from build123d import *

# Parameters (mm, degrees)
F1_DEPTH = 10
F2_R     = 1
F3_DEPTH = 6.2


# Not quite as in the source:
# - ends of sketch curves that miss each other by under 0.0002 mm in the source are joined


with BuildPart() as f1:
    # F0 (on Top) → F1 (new body)
    with BuildSketch(Plane.XY):
        with BuildLine():
            Line((-0.3999973293, 5), (-6.2999973293, 5))
            Line((-6.2999973293, 5), (-6.2999973293, -5))
            Line((-6.2999973293, -5), (6.3, -5))
            Line((6.3, -5), (6.3, 5))
            Line((6.3, 5), (0.4, 5))
            ThreePointArc((0.4, 5), (0.2585786438, 4.9414213562), (0.2, 4.8))
            Line((0.2, 4.8), (0.2, 0))
            ThreePointArc((0.2, 0), (0.1414213562, -0.1414213562), (0, -0.2))
            ThreePointArc((0, -0.2), (-0.1414186856, -0.1414213562), (-0.1999973293, 0))
            Line((-0.1999973293, 0), (-0.1999973293, 4.8))
            ThreePointArc((-0.1999973293, 4.8), (-0.2585759731, 4.9414213562), (-0.3999973293, 5))
        make_face()
    extrude(amount=F1_DEPTH)

    # F2 (on face) → F3 (cut)
    with BuildSketch(Plane(origin=(-6.2999973293, 0, 0), x_dir=(0, -1, 0), z_dir=(-1, 0, 0))):
        with Locations((-3, 5)):
            Circle(F2_R)
    extrude(amount=-F3_DEPTH, mode=Mode.SUBTRACT)


solid = f1.part
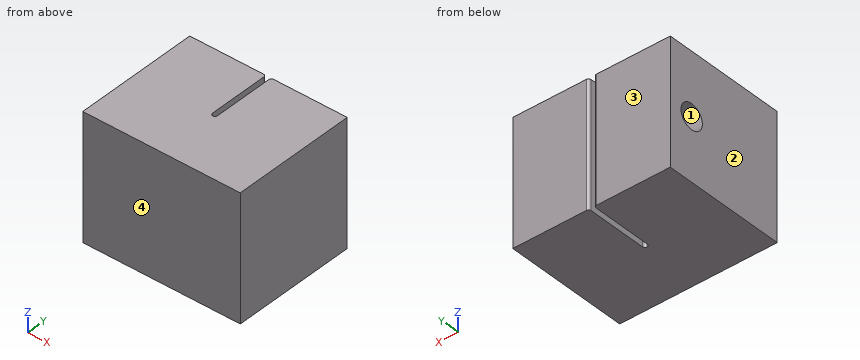
Could you check a few things on this model? Use its own coordinates, in mm. Face numbers are marked on the shaded views. Give positions to 0.01 mm unless a question says otherwise; leave off trailing zeros. Order: outer loops, then holes, each group sorted by start corner. A loop starts at its lowest first (then second) coordinate and runs counter-clockwise, first axis right, second up.
1. We'd pull the mould along Y, two halves only. Please class the marked faces 1, 2, 3 and 4: pulls with the +Y half, pulls with the -Y half, needs draft (parallel to the pull), parting line crosses it, or undercut.
2. I need wall thicknesses on L1, parallel to Z at x = -1.75, y = 3; L2, parallel to X at y = 2, z = 6; L3, parallel to X at y = 3.75, z = 4.75. Which ranges of each line are inside material? Lowest first, please.
3. Suppose I cut it at C-C (x = -1). List the corners of the cut face in (y, z) for me, plus the area to 3 significant figures.
4. Suppose I cut it at A-A (z = 5). List the corners of the cut face in (x, y) for me, plus the area to 3 significant figures.
5. Will these pins go through, and if not, where does the flat tip stop? P1, Ø1.6, axis at y = 3, z = 5, coming from the -X side; P2, Ø5, axis at y = 3, z = 5.5, coming from the -X side.
6. Suppose I cut it at B-B (y = 3). List the corners of the cut face in (x, z) for me, plus the area to 3 significant figures.
7. Suppose I cut it at D-D (z = 9). List the corners of the cut face in (x, y) for me.
Solved:
1. face 1: undercut
1. face 2: needs draft
1. face 3: pulls with the +Y half
1. face 4: pulls with the -Y half
2. L1: z = 0 to 4, 6 to 10
2. L2: x = -6.3 to -0.2, 0.2 to 6.3
2. L3: x = 0.2 to 6.3
3. outline: (-5, 0) - (5, 0) - (5, 10) - (-5, 10) - close; hole circle Ø2 at (3, 5)
3. area: 96.9 mm2
4. outline: (-6.3, -5) - (6.3, -5) - (6.3, 5) - (0.4, 5) arc R0.2 ccw to (0.2, 4.8) - (0.2, 0) arc R0.2 cw to (0, -0.2) arc R0.2 cw to (-0.2, 0) - (-0.2, 2) - (-6.3, 2) - close; (-6.3, 4) - (-0.2, 4) - (-0.2, 4.8) arc R0.2 ccw to (-0.4, 5) - (-6.3, 5) - close
4. area: 112 mm2
5. P1: stops at x = 0.2
5. P2: stops at x = -6.3
6. outline: (-6.3, 0) - (-0.2, 0) - (-0.2, 4) - (-6.3, 4) - close; (-6.3, 6) - (-0.2, 6) - (-0.2, 10) - (-6.3, 10) - close; (0.2, 0) - (6.3, 0) - (6.3, 10) - (0.2, 10) - close
6. area: 110 mm2
7. outline: (-6.3, -5) - (6.3, -5) - (6.3, 5) - (0.4, 5) arc R0.2 ccw to (0.2, 4.8) - (0.2, 0) arc R0.2 cw to (0, -0.2) arc R0.2 cw to (-0.2, 0) - (-0.2, 4.8) arc R0.2 ccw to (-0.4, 5) - (-6.3, 5) - close
